```python
from build123d import *

# Parameters (mm, degrees)
F1_DEPTH = 5
F2_R     = 5
F3_R     = 2.5
F4_DEPTH = 0.5


with BuildPart() as f1:
    # F0 (on Top) → F1 (new body)
    with BuildSketch(Plane.XY):
        Polygon((12.5, 75), (-12.5, 75), (-12.5, 21.650635), (-58.701905, 48.325318), (-71.201905, 26.674682), (-25, 0), (-71.201905, -26.674682), (-58.701905, -48.325318), (-12.5, -21.650635), (-12.5, -75), (12.5, -75), (12.5, -21.650635), (58.701905, -48.325318), (71.201905, -26.674682), (25, 0), (71.201905, 26.674682), (58.701905, 48.325318), (12.5, 21.650635), align=None)
    extrude(amount=F1_DEPTH)

    # F2
    f2_edges = [f1.edges().sort_by_distance(p)[0] for p in [
        (-71.201905, -26.674682, 2.5),
        (-58.701905, -48.325318, 2.5),
        (-12.5, -75, 2.5),
        (12.5, -75, 2.5),
        (-71.201905, 26.674682, 2.5),
        (58.701905, -48.325318, 2.5),
        (71.201905, -26.674682, 2.5),
        (71.201905, 26.674682, 2.5),
        (58.701905, 48.325318, 2.5),
        (12.5, 75, 2.5),
        (-12.5, 75, 2.5),
        (-58.701905, 48.325318, 2.5),
    ]]
    fillet(f2_edges, radius=F2_R)

    # F3 (on face) → F4 (cut)
    with BuildSketch(Plane.XY.offset(5)):
        with Locations((0, 65)):
            Circle(F3_R)
    extrude(amount=-F4_DEPTH, mode=Mode.SUBTRACT)


solid = f1.part
```
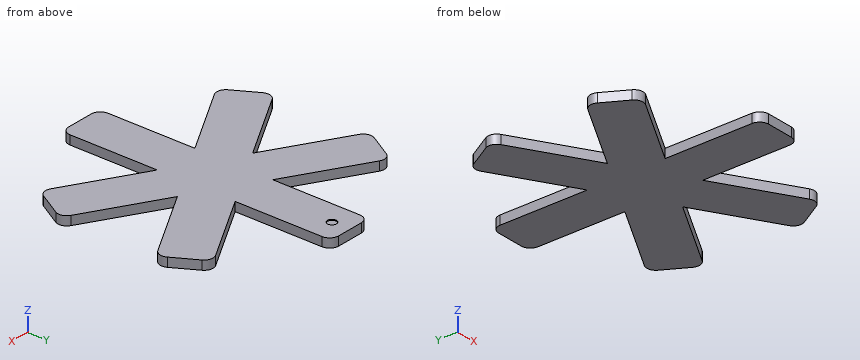
Can you work these out from the model? Positions are in its coordinate system, mm. Coordinates: 2 decimals unless noted, no trailing zeros. Loops run counter-clockwise (first coordinate to the right, second up) from the corner with the lowest first, then second, coordinate; pieces in that order, holes last.
Item 1: Suppose I cut it at B-B (y = 65). Please give me the cut outline in (x, z), then the cut area to 4 significant figures.
Answers below:
outline: (-12.5, 0) - (12.5, 0) - (12.5, 5) - (2.5, 5) - (2.5, 4.5) - (-2.5, 4.5) - (-2.5, 5) - (-12.5, 5) - close
area: 122.5 mm2
Item 2: Suppose I cut it at A-A (x = -36). Please give me the cut outline in (y, z), then the cut area to 3 significant figures.
Answers below:
outline: (-35.22, 0) - (-6.35, 0) - (-6.35, 5) - (-35.22, 5) - close; (6.35, 0) - (35.22, 0) - (35.22, 5) - (6.35, 5) - close
area: 289 mm2
Item 3: Suppose I cut it at D-D (y = 42). Please give me the cut outline in (x, z), then the cut area to 3 significant figures.
Answers below:
outline: (-62.35, 0) - (-47.75, 0) - (-47.75, 5) - (-62.35, 5) - close; (-12.5, 0) - (12.5, 0) - (12.5, 5) - (-12.5, 5) - close; (47.75, 0) - (62.35, 0) - (62.35, 5) - (47.75, 5) - close
area: 271 mm2
Item 4: Please list where these lines run through material, in increasing order: L1, parallel to Y at x = 0, z = 4.75; L2, parallel to X at y = 30, z = 4.35; L3, parallel to X at y = -53, z = 1.
Answers below:
L1: y = -75 to 62.5, 67.5 to 75
L2: x = -69.14 to -26.96, -12.5 to 12.5, 26.96 to 69.14
L3: x = -12.5 to 12.5
Item 5: I'm going to push flat-ended pins straight in: pin 1 (1.5 mm diameter, centred on y = 40, z = 2, fed in from -X); pin 2 (2.5 mm diameter, centred on x = 0, y = 64.5, fed in from +Z); pin 3 (2.5 mm diameter, centred on y = -37.5, z = 3.5, fed in from -X). Where does each tip first touch, or does it pass through?
Answers below:
pin 1: stops at x = -63.94
pin 2: stops at z = 4.5
pin 3: stops at x = -65.67
